Work out the finished part from the listing and answer in its coordinate system (mm). A direction names the side the tool comes from. Coordinates: 2 decimals unless noted, no trailing zeros. Write each loop counter-clockwise with the first axis right and the second up, starting at its lowest first coordinate (ties: lowest second). Pieces come first, ordered by that corner, then holes. Notation, with made-up numbers: M 42.5,20 L 66.5,20 A6 cw 66.5,31 Z; hole C 59,-24 d4. An arc over 180 degrees is marked long. Answer as CSV lines item,"result". Start each with the question number.
(1) Flat-ended cylindrical pins translate along their axes: P1, Ø10, axis at x = -18.5, y = 31.5, coming from the -Z side; P2, Ø1.2, axis at x = -20.5, z = -2, coming from the -Y side; P3, Ø2.5, axis at x = -13.5, z = -3, coming from the +Y side. Find the tip coordinate at first contact, or state that the pin passes through.
(2) For faces 1 (the flat face through (-4, 32, -3)), 2 (the cylindrical face through (-0.285, 20.301, -2.535)), determine the directions among +Z, -Z, +X, -X, +Y, -Y from which every point of the face is accessible in a straight line to the end or side of a thin tool.
(3) A cutting plane is placed at A-A on y = 7.5. Give the vertices of the cut face in (x, z).
(4) Find the intervals of material crossed by L1, parallel to Y at x = -10.5, z = -2.5; L2, parallel to X at y = 5, z = 3; L3, parallel to Y at x = -15.25, z = -2, in increasing order. Write a range as [from, to].
(5) A cutting plane is placed at D-D on x = -3.75. Give the vertices of the cut face in (y, z).
(6) The mould has two halves that part along Y. Classify faces 3 (the flat face through (-21, 28, -3)), 4 (the flat face through (-15.5, 13, -3)), 5 (the cylindrical face through (-15.199, 0.285, -2.591)): released by +Y, released by -Y, zero draft, split by the parting line, or undercut.
Autodesk Inventor part; units mm, degrees
ref_plane "YZ Plane" through (0, 0, 0) normal (1, 0, 0) x (0, 1, 0)
ref_plane "XZ Plane" through (0, 0, 0) normal (0, 1, 0) x (-1, 0, 0)
ref_plane "XY Plane" through (0, 0, 0) normal (0, 0, 1) x (1, 0, 0)
sketch "스케치1" plane through (0, 0, 0) normal (0, 1, 0) x (-1, 0, 0)
  point P0 (0, 0)
sketch "스케치2" plane through (0, 0, 0) normal (0, 1, 0) x (-1, 0, 0)
  line L0 (0, 0) -> (24, 0)
  line L1 (24, 0) -> (24, -5)
  line L2 (24, -5) -> (0, -5)
  line L3 (0, -5) -> (0, 0)
  dimension "d0" = 24
  dimension "d1" = 5
extrude "돌출1" add sketch "스케치2" along normal blind 25
sketch "스케치3" plane through (0, 25, 0) normal (0, 1, 0) x (1, 0, 0)
  line L0 (-21, 0) -> (-3, 0)
  line L1 (-3, 0) -> (-3, 5)
  line L2 (-3, 5) -> (-21, 5)
  line L3 (-21, 5) -> (-21, 0)
  line L4 (0, 5) -> (-24, 5)
  line L5 (-24, 0) -> (0, 0)
  line L6 (-24, 5) -> (-24, 0)
  line L7 (0, 0) -> (0, 5)
  dimension "d4" = 3
  dimension "d5" = 3
extrude "돌출2" add sketch "스케치3" along normal blind 11 contours L5 L6 L4 L3 | L1 L4 L7 L5
sketch "스케치4" plane through (-21, 25, 0) normal (1, 0, 0) x (0, 0, -1)
  line L0 (0, 0) -> (0, 11)
  line L1 (5, 11) -> (0, 11)
  line L2 (0, 11) -> (0, 7)
  line L3 (0, 7) -> (5, 7)
  line L4 (5, 7) -> (5, 11)
  point P0 (0, -25)
  dimension "d8" = 4
extrude "돌출3" add sketch "스케치4" along normal blind 1.5
sketch "스케치5" plane through (-3, 25, -5) normal (-1, 0, 0) x (0, 0, 1)
  line L0 (0, 11) -> (5, 11)
  line L1 (5, 11) -> (0, 11)
  line L2 (0, 11) -> (0, 7)
  line L3 (0, 7) -> (5, 7)
  line L4 (5, 7) -> (5, 11)
  point P0 (5, -25)
  dimension "d11" = 4
extrude "돌출4" add sketch "스케치5" along normal blind 1.5
sketch "스케치6" plane through (-24, 0, 0) normal (0, 0, 1) x (1, 0, 0)
  line L0 (0, 0) -> (24, 0)
  line L1 (0, 0) -> (0, 36)
  line L2 (24, 0) -> (0, 0)
  line L3 (0, 0) -> (0, 20)
  line L4 (0, 20) -> (24, 20)
  line L5 (24, 20) -> (24, 0)
  line L6 (3, 25) -> (21, 25)
  dimension "d14" = 5
extrude "돌출5" add sketch "스케치6" along normal blind 5
sketch "스케치7" plane through (0, 0, -5) normal (0, 0, -1) x (-1, 0, 0)
  line L0 (0, 20) -> (24, 20)
  line L1 (24, 20) -> (24, 0)
  line L2 (24, 0) -> (0, 0)
  line L3 (0, 0) -> (0, 20)
  line L4 (0, 0) -> (0, 36)
  line L5 (24, 0) -> (24, 36)
  line L6 (24, 0) -> (0, 0)
  line L7 (3, 25) -> (21, 25)
  dimension "d17" = 5
extrude "돌출6" add sketch "스케치7" along normal blind 5
sketch "스케치8" plane through (0, 36, 0) normal (1, 0, 0) x (0, 0, -1)
  line L0 (10, -16) -> (10, -36)
  line L1 (-5, -36) -> (-5, -16)
  point P0 (0, -36)
  dimension "d20" = 15
sketch "스케치9" plane through (-24, 36, -5) normal (-1, 0, 0) x (0, 0, 1)
  circle A0 centre (2.5, -28.5) radius 4.95
  line L0 (-5, -36) -> (-5, -16)
  line L1 (10, -36) -> (-5, -36)
  line L2 (0, 0) -> (5, 0)
  point P0 (5, -36)
  dimension "d21" = 9.9
  dimension "d22" = 7.5
  dimension "d23" = 7.5
  dimension "d24" = 36
sketch "스케치10" plane through (-24, 36, -5) normal (-1, 0, 0) x (0, 0, 1)
  line L0 (0, -16) -> (-5, -16)
  line L1 (-5, -36) -> (10, -36)
  line L2 (-5, -16) -> (10, -16)
  line L3 (10, -16) -> (10, -36)
  line L4 (10, -36) -> (-5, -36)
  line L5 (-5, -36) -> (-5, -16)
  circle A0 centre (2.5, -28.5) radius 4.95
  point P0 (5, -36)
extrude "돌출7" cut sketch "스케치10" against normal blind 50 contours A0
sketch "스케치11" plane through (-24, 36, -5) normal (-1, 0, 0) x (0, 0, 1)
  line L0 (0, -16) -> (-5, -16)
  line L1 (10, -16) -> (10, -36)
  line L2 (-5, -16) -> (10, -16)
  line L3 (10, -16) -> (10, -36)
  line L4 (10, -36) -> (-5, -36)
  line L5 (-5, -36) -> (-5, -16)
  point P0 (5, -36)
extrude "돌출8" cut sketch "스케치11" against normal blind 8.5
sketch "스케치12" plane through (0, 36, 0) normal (1, 0, 0) x (0, 0, -1)
  line L0 (0, -16) -> (-5, -16)
  line L1 (10, -36) -> (10, -16)
  line L2 (-5, -16) -> (10, -16)
  line L3 (10, -16) -> (10, -36)
  line L4 (10, -36) -> (-5, -36)
  line L5 (-5, -36) -> (-5, -16)
  point P0 (0, -36)
extrude "돌출9" cut sketch "스케치12" against normal blind 8.5
sketch "스케치13" plane through (-24, 0, 5) normal (0, 0, 1) x (1, 0, 0)
  point P0 (24, 0)
fillet "모깎기1" radius 4 4 edges at (-12, 20, 0) (-15.5, 20, -2.5) (-12, 20, -5) (-8.5, 20, -2.5)
fillet "모깎기2" radius 1 18 edges at (-8.5, 10, -10) (-8.5, 10, 5) (-8.5, 0, -2.5) (-15.5, 10, -10) (-12, 20, -10) (-12, 20, 5) (-15.5, 10, 5) (-15.5, 0, -2.5) (-12, 0, 5) (-12, 0, -10) (0, 20, -2.5) (0, 36, -2.5) (0, 28, -5) (0, 28, 0) (-24, 28, 0) (-24, 28, -5) (-24, 20, -2.5) (-24, 36, -2.5)
fillet "모깎기3" radius 3.5 2 edges at (-4.5, 36, -2.5) (-19.5, 36, -2.5)
sketch "스케치14" plane through (-3, 25, -5) normal (0, 0, -1) x (-1, 0, 0)
  line L0 (18, 7) -> (18, 0)
  line L1 (0, 0) -> (0, 7)
  point P0 (-3, -25)
  dimension "d34" = 18
sketch "스케치15" plane through (-21, 25, 0) normal (0, 0, 1) x (1, 0, 0)
  line L0 (0, 7) -> (1.5, 7)
  line L1 (0, 0) -> (18, 0)
  point P0 (21, -25)
  dimension "d35" = 7
sketch "스케치16" plane through (-24, 0, 5) normal (0, 0, 1) x (1, 0, 0)
  line L0 (14.5, 19) -> (14.5, 1)
  line L1 (9.5, 1) -> (9.5, 19)
  point P0 (24, 0)
  dimension "d36" = 5
sketch "스케치17" plane through (-8.5, 36, 0) normal (1, 0, 0) x (0, 0, -1)
  point P0 (0, -36)
properties part number "보조바퀴 축"
Here are the results:
1,P1,"stops at z = -5"
1,P2,"stops at y = 20"
1,P3,"stops at y = 25"
2,face 1,"+Z, -Z"
2,face 2,"+Z, -Z, +X, -Y"
3,outline,"M -15.5,-9 A1 ccw -14.5,-10 L -9.5,-10 A1 ccw -8.5,-9 L -8.5,-7.45 L -15.5,-7.45 Z; M -15.5,2.45 L -8.5,2.45 L -8.5,4 A1 ccw -9.5,5 L -14.5,5 A1 ccw -15.5,4 Z"
4,L1,"y = [0, 2.55], [12.45, 25]"
4,L2,"x = [-15.5, -8.5]"
4,L3,"y = [0.34, 2.58], [12.42, 25]"
5,outline,"M 20,-5 L 25,-5 L 25,0 L 20,0 Z; M 32,-5 L 34.67,-5 L 34.67,0 L 32,0 Z"
6,face 3,"undercut"
6,face 4,"zero draft"
6,face 5,"released by -Y"
